Check sheet for the drawn part. Datum: minimum x, y, z corner. Units: mm. Round coordinates to 2 decimals unless told otherwise and drop trailing zeros. Loops run counter-clockwise (first coordinate to the right, second up) from the corner with the lowest first, then second, coordinate; pieces in that order, holes last.
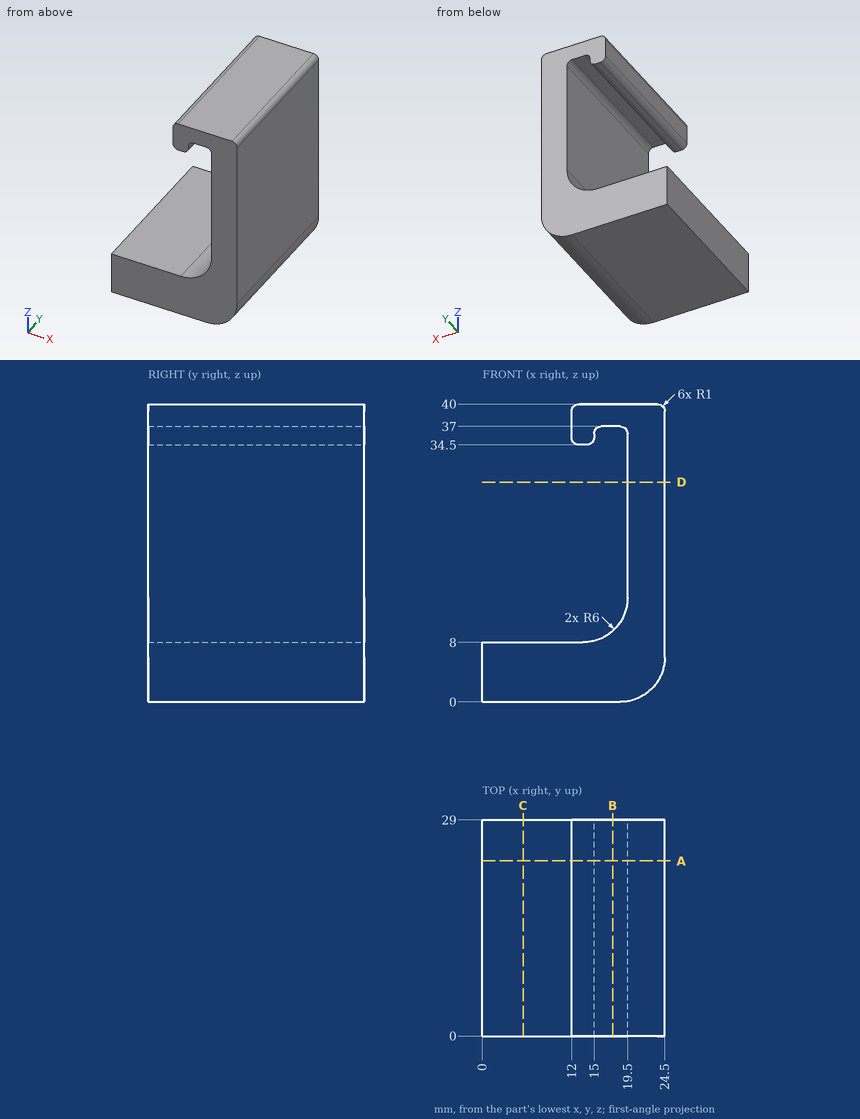
1. Section check B-B (x = 17.5). Enter the section's corners in (y, z), then the cut area to 3 significant figures.
2. Scan lines: L1, parallel to Z at x = 3.25, y = 17.75; L2, parallel to X at y = 3.5, z = 29; L3, parallel to Z at x = 13.5, y = 6.5. Record each from-to range of solid material in increasing order.
3. Section check C-C (x = 5.5). Enter the section's corners in (y, z).
4. Gauge pin test, flat ends, axial feed: P1, Ø7, axis at x = 4, y = 16.5, coming from the +Z side; P2, Ø4, axis at y = 9.5, z = 36.5, coming from the -X side. Record the tip position at first contact, or that the pin passes through.
5. Section check A-A (y = 23.5). Enter the section's corners in (x, z), then the cut area to 3 significant figures.
6. Section check D-D (z = 29.5). Enter the section's corners in (x, y).
Taken from the geometry:
1. outline: (0, 0) - (29, 0) - (29, 9.53) - (0, 9.53) - close; (0, 37) - (29, 37) - (29, 40) - (0, 40) - close
1. area: 363 mm2
2. L1: z = 0 to 8
2. L2: x = 19.5 to 24.5
2. L3: z = 0 to 8, 34.5 to 40
3. outline: (0, 0) - (29, 0) - (29, 8) - (0, 8) - close
4. P1: stops at z = 8
4. P2: stops at x = 12
5. outline: (0, 0) - (18.5, 0) arc R6 ccw to (24.5, 6) - (24.5, 39) arc R1 ccw to (23.5, 40) - (13, 40) arc R1 ccw to (12, 39) - (12, 35.5) arc R1 ccw to (13, 34.5) - (14, 34.5) arc R1 ccw to (15, 35.5) - (15, 36) arc R1 cw to (16, 37) - (18.5, 37) arc R1 cw to (19.5, 36) - (19.5, 14) arc R6 cw to (13.5, 8) - (0, 8) - close
5. area: 386 mm2
6. outline: (19.5, 0) - (24.5, 0) - (24.5, 29) - (19.5, 29) - close
